Verification items for the finished model (mm, model axes). Face numbers are marked on the shaded views. A direction names the side the tool comes from. Give positions to 0.01 mm unless a question says otherwise; leave off trailing zeros. Loops run counter-clockwise (first coordinate to the right, second up) from the corner with the lowest first, then second, coordinate; pieces in that order, holes last. Notation, with made-up numbers: (57.25, -28) - (86.25, -28) arc R15 ccw to (86.25, -20) - close; hole circle Ø2 at (15, 73). An arc over 180 degrees is marked (long way). One line per question, with ' | ' between items. Start each with the question number.
1. Section check B-B, the plane z = 40.5. Enter the section's corners in (x, y), then the cut area to 3 significant figures.
2. Depth check by flat-ended pin: pin 1 Ø0.5 at (x, y) = (48.5, 36) entering from +Z; pin 2 Ø5 at (y, z) = (37, 59) entering from -X; pin 3 Ø3 at (y, z) = (39, 59) entering from +X. Enter the tip coordinate at first touch or a pass-through.
3. Section check C-C, the plane y = 40.5. Enter the section's corners in (x, z), then the cut area to 3 significant figures.
4. Section check D-D, the plane x = -4. Enter the section's corners in (y, z), then the cut area to 3 significant figures.
5. Section check A-A, the plane x = 10.5. Enter the section's corners in (y, z).
6. Thickness scan on line 1 along Y through (x, z) = (29, 61.25); line 2 along Z through (x, y) = (20, 35.5); line 3 along Y through (x, z) = (4.5, 56.5). Record the ranges inside material, lowest first. Write a range as from..to.
7. Tool access check on the marked faces 1, 2 and 3. Record the directions out of +Z, -Z, +X, -X, +Y, -Y that give a thin tool (end or side, any length) a straight path to the whole face; none if there is none.
from build123d import *

# Parameters (mm, degrees)
COMBINE1_START     = 34.612659565
COMBINE1_DEPTH     = 2
COMBINE1_START_2   = 37.615879947
COMBINE1_2_DEPTH   = 25.5
COMBINE1_START_3   = 36.615879947
COMBINE1_3_DEPTH   = 27.5
CUT_EXTRUDE1_DEPTH = 0.5
CUT_EXTRUDE2_DEPTH = 0.5
CUT_EXTRUDE3_DEPTH = 0.5
CUT_EXTRUDE5_DEPTH = 0.5
SKETCH9_W          = 5
SKETCH9_H          = 24.5
CUT_EXTRUDE6_DEPTH = 1
SKETCH10_W         = 40
SKETCH10_H         = 2
CUT_EXTRUDE7_DEPTH = 1


with BuildPart() as part:
    # Combine1: read off the stored shape, not the designer's step
    # Combine1 outline → Combine1 (new body)
    with BuildSketch(Plane(origin=(0, 0, 0), x_dir=(1, 0, 0), z_dir=(0, 1, 0)).offset(COMBINE1_START)):
        Polygon((17.883282848, -59.365879947), (27.883282848, -59.365879947), (27.883282848, -61.115879947), (28.327718217, -61.115879947), (29.146651244, -63.365879947), (29.761507101, -63.365879947), (30.580440128, -61.115879947), (31.469310867, -61.115879947), (32.288243894, -63.365879947), (32.903099751, -63.365879947), (33.722032778, -61.115879947), (34.610903517, -61.115879947), (35.429836544, -63.365879947), (36.044692401, -63.365879947), (36.863625428, -61.115879947), (37.752496167, -61.115879947), (38.571429194, -63.365879947), (39.186285051, -63.365879947), (40.005218078, -61.115879947), (40.894088817, -61.115879947), (41.713021844, -63.365879947), (42.327877701, -63.365879947), (43.146810728, -61.115879947), (44.035681467, -61.115879947), (44.854614494, -63.365879947), (45.469470351, -63.365879947), (46.288403378, -61.115879947), (47.177274117, -61.115879947), (47.996207144, -63.365879947), (48.611063001, -63.365879947), (49.429996028, -61.115879947), (50.318866767, -61.115879947), (51.137799794, -63.365879947), (51.752655651, -63.365879947), (52.571588678, -61.115879947), (53.460459417, -61.115879947), (54.279392444, -63.365879947), (54.894248301, -63.365879947), (55.713181328, -61.115879947), (56.602052067, -61.115879947), (57.420985094, -63.365879947), (57.883282848, -63.365879947), (57.883282848, -50.365879947), (17.883282848, -50.365879947), align=None)
    extrude(amount=COMBINE1_DEPTH)

    # Combine1 2 outline → Combine1 2 (add)
    with BuildSketch(Plane.XY.offset(COMBINE1_START_2)):
        Polygon((17.883282848, 44.075659565), (15.882661668, 44.075659565), (-10.116717152, 34.612659565), (17.883282848, 34.612659565), align=None)
    extrude(amount=COMBINE1_2_DEPTH)

    # Combine1 3 outline → Combine1 3 (add)
    with BuildSketch(Plane.XY.offset(COMBINE1_START_3)):
        Polygon((17.883282848, 38.612659565), (0.873192525, 38.612659565), (-4.621762313, 36.612659565), (17.883282848, 36.612659565), align=None)
    extrude(amount=COMBINE1_3_DEPTH)

    # Sketch2 → Cut-Extrude1 (cut)
    with BuildSketch(Plane.XY.offset(63.115879947)):
        Polygon((0.873192525, 38.612659565), (15.882661668, 44.075659565), (17.883282848, 44.075659565), (17.883282848, 38.612659565), align=None)
        Polygon((17.883282848, 36.612659565), (17.883282848, 34.612659565), (-10.116717152, 34.612659565), (-4.621762313, 36.612659565), align=None)
    extrude(amount=-CUT_EXTRUDE1_DEPTH, mode=Mode.SUBTRACT)

    # Sketch3 → Cut-Extrude2 (cut)
    with BuildSketch(Plane.XY.offset(64.115879947)):
        Polygon((17.883282848, 36.612659565), (17.883282848, 38.612659565), (0.873192525, 38.612659565), (-4.621762313, 36.612659565), align=None)
    extrude(amount=-CUT_EXTRUDE2_DEPTH, mode=Mode.SUBTRACT)

    # Sketch4 → Cut-Extrude3 (cut)
    with BuildSketch(Plane(origin=(0, 0, 37.615879947), x_dir=(-1, 0, 0), z_dir=(0, 0, -1))):
        Polygon((-17.883282848, 38.612659565), (-17.883282848, 44.075659565), (-15.882661668, 44.075659565), (-0.873192525, 38.612659565), align=None)
        Polygon((-17.883282848, 36.612659565), (4.621762313, 36.612659565), (10.116717152, 34.612659565), (-17.883282848, 34.612659565), align=None)
    extrude(amount=-CUT_EXTRUDE3_DEPTH, mode=Mode.SUBTRACT)

    # Sketch7 → Cut-Extrude5 (cut)
    with BuildSketch(Plane(origin=(0, 0, 36.615879947), x_dir=(-1, 0, 0), z_dir=(0, 0, -1))):
        Polygon((-17.883282848, 38.612659565), (-17.883282848, 36.612659565), (4.621762313, 36.612659565), (-0.873192525, 38.612659565), align=None)
    extrude(amount=-CUT_EXTRUDE5_DEPTH, mode=Mode.SUBTRACT)

    # Sketch9 → Cut-Extrude6 (cut)
    with BuildSketch(Plane(origin=(0, 44.075659565, 0), x_dir=(1, 0, 0), z_dir=(0, 1, 0))):
        with Locations((15.383282848, -50.365879947)):
            Rectangle(SKETCH9_W, SKETCH9_H)
    extrude(amount=-CUT_EXTRUDE6_DEPTH, mode=Mode.SUBTRACT)

    # Sketch10 → Cut-Extrude7 (cut)
    with BuildSketch(Plane(origin=(0, 0, 50.365879947), x_dir=(-1, 0, 0), z_dir=(0, 0, -1))):
        with Locations((-37.883282848, 35.612659565)):
            Rectangle(SKETCH10_W, SKETCH10_H)
    extrude(amount=-CUT_EXTRUDE7_DEPTH, mode=Mode.SUBTRACT)


solid = part.part
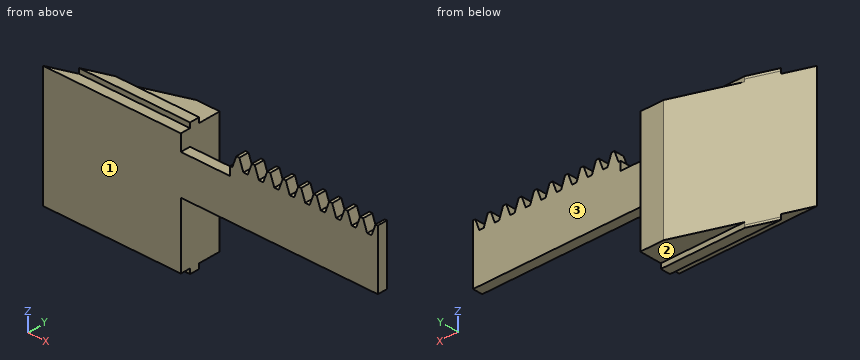
Results list:
1) outline: (-10.12, 34.61) - (17.88, 34.61) - (17.88, 43.08) - (13.14, 43.08) - close | area: 139 mm²
2) pin 1: z = 63.37 | pin 2: x = -10.12 | pin 3: x = 17.88
3) outline: (6.06, 38.12) - (17.88, 38.12) - (17.88, 62.62) - (6.06, 62.62) - close | area: 290 mm²
4) outline: (34.61, 38.12) - (36.61, 38.12) - (36.61, 37.12) - (36.84, 37.12) - (36.84, 63.62) - (36.61, 63.62) - (36.61, 62.62) - (34.61, 62.62) - close | area: 55.0 mm²
5) outline: (34.61, 38.12) - (36.61, 38.12) - (36.61, 37.12) - (38.61, 37.12) - (38.61, 38.12) - (42.12, 38.12) - (42.12, 62.62) - (38.61, 62.62) - (38.61, 63.62) - (36.61, 63.62) - (36.61, 62.62) - (34.61, 62.62) - close
6) line 1: 34.61..36.61 | line 2: 51.37..59.37 | line 3: 34.61..39.93
7) face 1: +Z, -Z, +X, -X, -Y | face 2: -Z, +X, -X, +Y | face 3: +Z, -Z, +X, +Y
